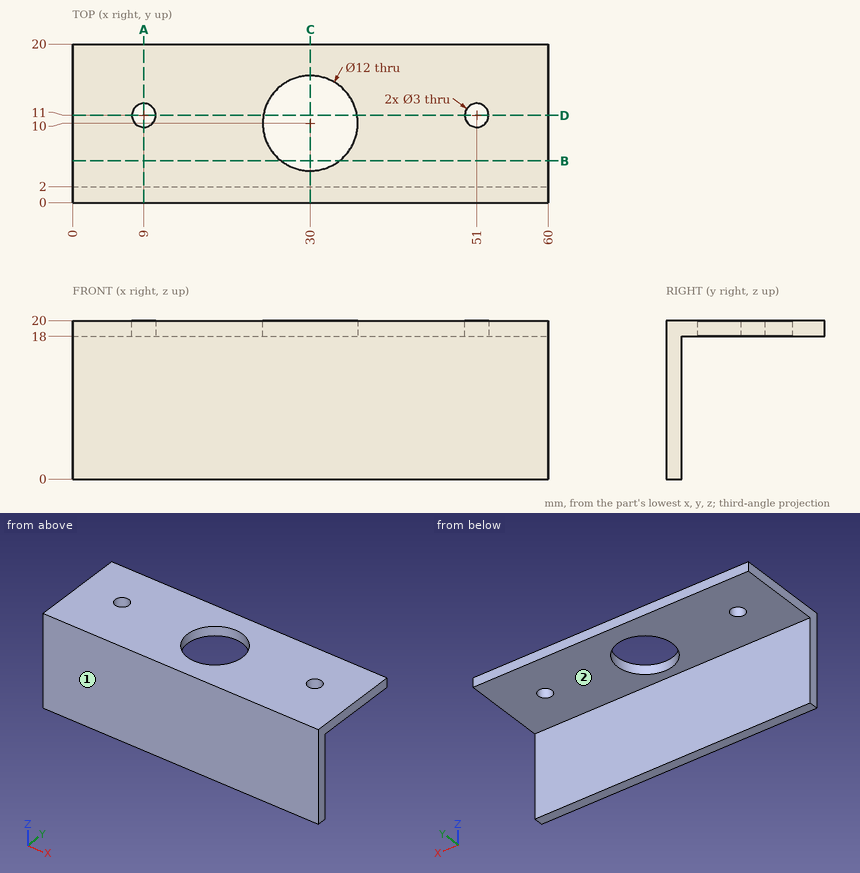
Verification items for this drawing (mm, ordinates from the low corner). A direction names the side the tool comes from. Round coordinates to 2 decimals unless told otherwise and drop trailing zeros. Write each loop counter-clockwise with the first axis right and the second up, starting at its lowest first coordinate (ties: lowest second). Pieces come first, ordered by that corner, then holes. Notation, with made-up numbers: (13, 36.25) - (44, 36.25) arc R24 cw to (44, 73.25) - close; hole circle Ø4 at (49.5, 21.25). An arc over 180 degrees is marked (long way). Answer as a JSON object with one key per item and string values. Group by question number.
Q1. Section check B-B, the plane y = 5.25. Enter the section's corners in (x, z).
Q2. Tool access check on the marked faces 1 and 2. Record the directions out of +Z, -Z, +X, -X, +Y, -Y that give a thin tool (end or side, any length) a straight path to the whole face; none if there is none.
Q3. Go/stop test with flat-tipped pins: pin 1 Ø4 at (x, z) = (17.5, 4) entering from +Y; pin 2 Ø5 at (x, z) = (18, 11) entering from -Y; pin 3 Ø4 at (y, z) = (4.5, 15) entering from -X; pin 4 Ø5 at (x, y) = (51, 11) entering from -Z. Record where each tip stops, or that it passes through.
Q4. Section check A-A, the plane x = 9. Enter the section's corners in (y, z).
Q5. Section check C-C, the plane x = 30. Enter the section's corners in (y, z), plus the area to 3 significant figures.
Q6. Section check D-D, the plane y = 11. Enter the section's corners in (x, z).
Q7. Thickness scan on line 1 (Y direction, x = 30, z = 19); line 2 (Y direction, x = 9, z = 19.05); line 3 (Y direction, x = 46.5, z = 9). Record the ranges inside material, lowest first.
Found:
{
 "1": {"outline": "(0, 18) - (26.33, 18) - (26.33, 20) - (0, 20) - close; (33.67, 18) - (60, 18) - (60, 20) - (33.67, 20) - close"},
 "2": {"face 1": "+Z, -Z, +X, -X, -Y", "face 2": "-Z, +X, -X, +Y"},
 "3": {"pin 1": "stops at y = 2", "pin 2": "stops at y = 0", "pin 3": "passes through", "pin 4": "stops at z = 18"},
 "4": {"outline": "(0, 0) - (2, 0) - (2, 18) - (9.5, 18) - (9.5, 20) - (0, 20) - close; (12.5, 18) - (20, 18) - (20, 20) - (12.5, 20) - close"},
 "5": {"outline": "(0, 0) - (2, 0) - (2, 18) - (4, 18) - (4, 20) - (0, 20) - close; (16, 18) - (20, 18) - (20, 20) - (16, 20) - close", "area": "52.0 mm^2"},
 "6": {"outline": "(0, 18) - (7.5, 18) - (7.5, 20) - (0, 20) - close; (10.5, 18) - (24.08, 18) - (24.08, 20) - (10.5, 20) - close; (35.92, 18) - (49.5, 18) - (49.5, 20) - (35.92, 20) - close; (52.5, 18) - (60, 18) - (60, 20) - (52.5, 20) - close"},
 "7": {"line 1": "y = 0 to 4, 16 to 20", "line 2": "y = 0 to 9.5, 12.5 to 20", "line 3": "y = 0 to 2"}
}
